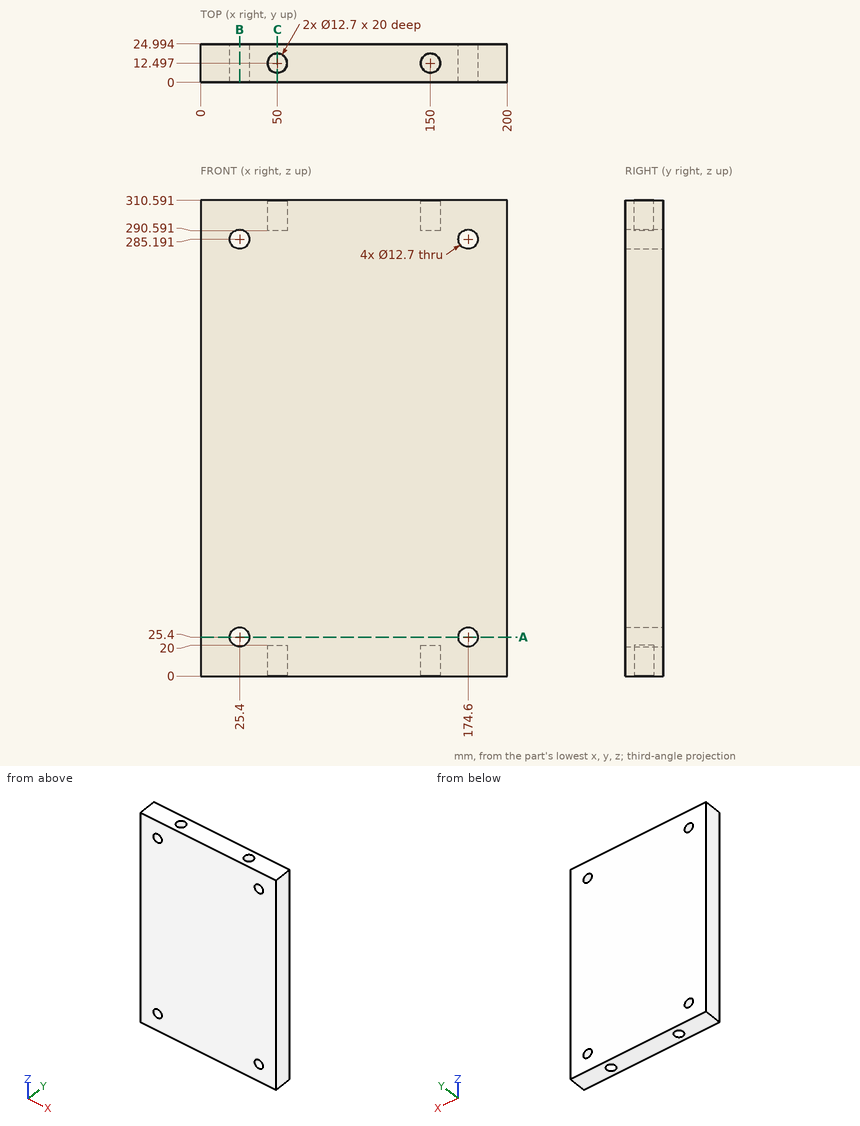
Geometry: see drawing. Coordinates: mm, zero at the bounding-box minimum. Coordinates: 2 decimals unless noted, no trailing zeros. Loops run counter-clockwise (first coordinate to the right, second up) from the corner with the lowest first, then second, coordinate; pieces in that order, holes last. Notation, with made-up numbers: M -10,19 L 32,19 A26 ccw 32,47 Z; hole C -32.75,-40 d11. An arc over 180 degrees is marked long. Answer in a Markdown table with one row per item.
Q1. Section C-C on x = 50. Return the cut outline in (y, z).
Answers below:
| item | result |
|---|---|
| outline | M 0,0 L 6.15,0 L 6.15,20 L 18.85,20 L 18.85,0 L 24.99,0 L 24.99,310.59 L 18.85,310.59 L 18.85,290.59 L 6.15,290.59 L 6.15,310.59 L 0,310.59 Z |
Q2. First-contact query: pin 1 (7.5 mm diameter, centred on x = 150, y = 12.5, fed in from -Z); pin 2 (10 mm diameter, centred on x = 48.5, y = 13, fed in from +Z). Flat tips, straight axial feed; report the tip coordinate or a pass-through.
Answers below:
| item | result |
|---|---|
| pin 1 | stops at z = 20 |
| pin 2 | stops at z = 310.59 |
Q3. Ray query, probe 1 along Z at (x, y) = (25.4, 13.5); probe 2 along Y at (x, z) = (50, 13.5); probe 3 along X at (y, z) = (7.75, 22) (1 decimal). Return the intervals inside material, ascending. Write a range as from..to.
Answers below:
| item | result |
|---|---|
| probe 1 | z = 0..19.05, 31.75..278.84, 291.54..310.59 |
| probe 2 | y = 0..6.15, 18.85..24.99 |
| probe 3 | x = 0..20, 30.8..169.2, 180..200 |
Q4. Section A-A on z = 25.4. Return the cut outline in (x, y).
Answers below:
| item | result |
|---|---|
| outline | M 0,0 L 19.05,0 L 19.05,24.99 L 0,24.99 Z; M 31.75,0 L 168.25,0 L 168.25,24.99 L 31.75,24.99 Z; M 180.95,0 L 200,0 L 200,24.99 L 180.95,24.99 Z |
Q5. Section B-B on x = 25.4. Return the cut outline in (y, z).
Answers below:
| item | result |
|---|---|
| outline | M 0,0 L 24.99,0 L 24.99,19.05 L 0,19.05 Z; M 0,31.75 L 24.99,31.75 L 24.99,278.84 L 0,278.84 Z; M 0,291.54 L 24.99,291.54 L 24.99,310.59 L 0,310.59 Z |
